Input: part model. Units: mm. Frame: model coordinates. Coordinates: 2 decimals unless noted, no trailing zeros. Loops run counter-clockwise (first coordinate to the right, second up) from the corner with the lowest first, then second, coordinate; pieces in that order, holes last.
Item 1: Section C-C on x = -17. Return loops of the section in (y, z) (3 decimals).
Item 2: Ray query, line 1 along Y through (x, z) = (-62, 4.5) (3 decimals); line 2 along X through (y, z) = (6, 3.5); line 3 along Y through (x, z) = (-57, 2). Return the intervals inside material, ascending.
Item 3: Contact query for flat-ended pins moving along their axis: P1, Ø3, axis at x = -13, z = 1.5, coming from the +Y side; P2, Ø1, axis at y = 27.5, z = 3.5, coming from the +X side. Output: stop coordinate, or through.
Item 4: Section B-B on y = 11. Return loops of the section in (x, z) (3 decimals).
Item 5: Pull-direction query (Y, two-part tool) for faces 1 (the flat face through (-29, 0, 5)), 2 (the cylindrical face through (-66.8, 28.55, 4.35)), 3 (the flat face through (-56, -4, 0)); classes: released by +Y, released by -Y, zero draft, split by the parting line, or undercut.
Autodesk Inventor part; units mm, degrees
ref_plane "YZ Plane" through (0, 0, 0) normal (1, 0, 0) x (0, 1, 0)
ref_plane "XZ Plane" through (0, 0, 0) normal (0, 1, 0) x (-1, 0, 0)
ref_plane "XY Plane" through (0, 0, 0) normal (0, 0, 1) x (1, 0, 0)
sketch "Sketch1" plane through (0, 0, 0) normal (0, 0, 1) x (1, 0, 0)
  line L0 (-57.15, 34.925) -> (-76.2, 34.925)
  line L1 (-76.2, 34.925) -> (-76.2, -12.7)
  line L2 (-76.2, -12.7) -> (0, -12.7)
  line L3 (0, -12.7) -> (0, 0)
  line L4 (0, 0) -> (-57.15, 0)
  line L5 (-57.15, 0) -> (-57.15, 34.925)
extrude "Extrusion1" add sketch "Sketch1" along normal blind 9.525
chamfer "Chamfer4" distance 2.54 angle 45 3 edges at (0, 0, 4.7625) (0, -6.35, 9.525) (0, -6.35, 0)
chamfer "Chamfer2" distance 0.381 angle 45 12 edges at (-76.2, 34.925, 4.7625) (-57.15, 34.925, 4.7625) (-57.15, 17.4625, 9.525) (-66.675, 34.925, 9.525) (-66.675, 34.925, 0) (-76.2, 11.1125, 9.525) (-76.2, 11.1125, 0) (-29.845, 0, 9.525) (-29.845, 0, 0) (-39.37, -12.7, 9.525) (-76.2, -12.7, 4.7625) (-39.37, -12.7, 0)
sketch "Sketch2" plane through (-76.2, -12.319, 0.381) normal (-1, 0, 0) x (0, 0, 1)
  circle A0 centre (4.3815, 37.719) radius 3.175
  line L0 (-0.381, 46.863) -> (-0.381, 0)
  line L1 (8.763, 47.244) -> (0, 47.244)
  dimension "d6" = 4.7625
  dimension "d7" = 9.525
extrude "Extrusion2" cut sketch "Sketch2" against normal through all
chamfer "Chamfer3" distance 0.381 angle 45 2 edges at (-57.15, 25.4, 1.5875) (-76.2, 25.4, 1.5875)
properties part number "index finger"
Results found:
1. outline: (-12.7, 0.381) - (-12.319, 0) - (-0.381, 0) - (0, 0.381) - (0, 9.144) - (-0.381, 9.525) - (-12.319, 9.525) - (-12.7, 9.144) - close
2. line 1: y = -12.7 to 22.236, 28.564 to 34.925
2. line 2: x = -76.2 to -57.15
2. line 3: y = -12.7 to 0
3. P1: stops at y = 0
3. P2: passes through
4. outline: (-76.2, 0.381) - (-75.819, 0) - (-57.15, 0) - (-57.15, 9.144) - (-57.531, 9.525) - (-75.819, 9.525) - (-76.2, 9.144) - close
5. face 1: released by +Y
5. face 2: undercut
5. face 3: zero draft
